```python
from build123d import *

# Parameters (mm, degrees)
SKETCH_1_W          = 20
SKETCH_1_H          = 20
EXTRUDE_1_DEPTH     = 25
SKETCH_2_W          = 20
SKETCH_2_H          = 11.5
CUT_EXTRUDE_1_DEPTH = 5
SKETCH_3_R          = 1.25
CUT_EXTRUDE_2_DEPTH = 25.494897428
SKETCH_4_R          = 1.25
CUT_EXTRUDE_3_DEPTH = 34.541019662
CHAMFER_1_SIZE      = 1
SKETCH_6_R          = 3.5
CUT_EXTRUDE_4_DEPTH = 4


with BuildPart() as part:
    # 草图1 → 凸台-拉伸1 (new body)
    with BuildSketch(Plane(origin=(0, 0, 0), x_dir=(0, 0, -1), z_dir=(1, 0, 0))):
        Rectangle(SKETCH_1_W, SKETCH_1_H)
    extrude(amount=EXTRUDE_1_DEPTH)

    # 草图2 → 切除-拉伸1 (cut)
    with BuildSketch(Plane.ZY):
        Rectangle(SKETCH_2_W, SKETCH_2_H)
    extrude(amount=-CUT_EXTRUDE_1_DEPTH, mode=Mode.SUBTRACT)

    # 草图3 → 切除-拉伸2 (cut, through all)
    with BuildSketch(Plane.ZY.offset(-5)):
        with Locations((-5, 0)):
            Circle(SKETCH_3_R)
        with Locations((5, 0)):
            Circle(SKETCH_3_R)
    extrude(amount=-CUT_EXTRUDE_2_DEPTH, mode=Mode.SUBTRACT)

    # 草图4 → 切除-拉伸3 (cut, through all)
    with BuildSketch(Plane(origin=(0, 10, 0), x_dir=(1, 0, 0), z_dir=(0, 1, 0))):
        with Locations(Location((20, 0, 0), (0, 0, 270))):
            Circle(SKETCH_4_R)
        with Locations(Location((10, 0, 0), (0, 0, 270))):
            Circle(SKETCH_4_R)
    extrude(amount=-CUT_EXTRUDE_3_DEPTH, mode=Mode.SUBTRACT)

    # 倒角1
    chamfer_1_edges = [part.edges().sort_by_distance(p)[0] for p in [
        (25, 0, -10),
        (25, 0, 10),
        (12.5, 10, 10),
        (12.5, 10, -10),
        (12.5, -10, -10),
        (12.5, -10, 10),
    ]]
    chamfer(chamfer_1_edges, length=CHAMFER_1_SIZE)

    # 草图6 → 切除-拉伸4 (cut)
    with BuildSketch(Plane(origin=(25, 0, 0), x_dir=(0, 0, -1), z_dir=(1, 0, 0))):
        with Locations((-5, 0)):
            Circle(SKETCH_6_R)
        with Locations((5, 0)):
            Circle(SKETCH_6_R)
    extrude(amount=-CUT_EXTRUDE_4_DEPTH, mode=Mode.SUBTRACT)


solid = part.part
```
Build history of the part. All positions in model axes, mm. A direction names the side the tool comes from. Coordinates: 2 decimals unless noted, no trailing zeros. Order: outer loops, then holes, each group sorted by start corner. A loop starts at its lowest first (then second) coordinate and runs counter-clockwise, first axis right, second up. Notation, with made-up numbers: (64.25, 11) -> (114.25, 11) arc R14 cw to (114.25, 18) -> close; hole circle Ø11 at (58, 86.5). An arc over 180 degrees is marked (long way). Answer in a Markdown table with one row per item. Add a question column.
Q1. Band-saw the part on A-A, the plane x = 20. List the corners of the cut face in (y, z), then the cut area to 3 significant figures.
Q2. Mould opens along Y. For faces 1 (the face through (12.3, -9.5, -9.5)), 2 (the face through (23.03, 1.05, -8.34)), 3 (the face through (25, 0, 0)) say: +Y half, -Y half, draft (parallel to the pull), parting line (faces both ways), or undercut.
Q3. Band-saw the part on C-C, the plane x = 3. List the corners of the cut face in (y, z).
Q4. Which spindle directions (+Z, -Z, +X, -X, +Y, -Y) get a long thin tool onto all of the face, cutting with end or side? Do faces 4 (the face through (12, 10, 0)), 5 (the face through (5, 0, 0)). Say none if no direction does.
Q5. Drop flat-ended pins along their axis: pin 1 (1.5 mm diameter, centred on y = -2, z = 7, fed in from +X); pin 2 (3 mm diameter, centred on y = 0, z = -5, fed in from +X); pin 3 (2 mm diameter, centred on x = 10, z = 0, fed in from +Y); pin 4 (4 mm diameter, centred on y = -3, z = -4.5, fed in from -X). Give the stop position or say it passes through.
Q6. Wall check: line 1 along X through (y, z) = (2.75, 0); line 2 along Y through (x, z) = (22.25, 5); line 3 along Z through (x, y) = (10.75, -0.25). Give the ranges that are in metal, low to high. Write a range as [from, to].
Q7. Band-saw the part on D-D, the plane z = -5. List the corners of the cut face in (x, y).
Q8. Band-saw the part on B-B, the plane y = 0. List the corners of the cut face in (x, z), then the cut area to 3 significant figures.
Answers follow:
| question | item | result |
|---|---|---|
| 1 | outline | (-10, -9) -> (-9, -10) -> (9, -10) -> (10, -9) -> (10, -1.25) -> (-10, -1.25) -> close; (-10, 1.25) -> (10, 1.25) -> (10, 9) -> (9, 10) -> (-9, 10) -> (-10, 9) -> close; hole circle Ø2.5 at (0, -5); hole circle Ø2.5 at (0, 5) |
| 1 | area | 338 mm^2 |
| 2 | face 1 | -Y half |
| 2 | face 2 | undercut |
| 2 | face 3 | draft |
| 3 | outline | (-10, -9) -> (-9, -10) -> (-5.75, -10) -> (-5.75, 10) -> (-9, 10) -> (-10, 9) -> close; (5.75, -10) -> (9, -10) -> (10, -9) -> (10, 9) -> (9, 10) -> (5.75, 10) -> close |
| 4 | face 4 | +Z, -Z, +X, -X, +Y |
| 4 | face 5 | +Z, -Z, -X |
| 5 | pin 1 | x = 25 |
| 5 | pin 2 | x = 21 |
| 5 | pin 3 | through |
| 5 | pin 4 | x = 5 |
| 6 | line 1 | [5, 8.75], [11.25, 18.75], [21.25, 25] |
| 6 | line 2 | [-10, -3.5], [3.5, 10] |
| 6 | line 3 | [-10, -6.22], [-3.78, -1], [1, 3.78], [6.22, 10] |
| 7 | outline | (0, -10) -> (25, -10) -> (25, -3.5) -> (21, -3.5) -> (21, -1.25) -> (5, -1.25) -> (5, -5.75) -> (0, -5.75) -> close; (0, 5.75) -> (5, 5.75) -> (5, 1.25) -> (21, 1.25) -> (21, 3.5) -> (25, 3.5) -> (25, 10) -> (0, 10) -> close |
| 8 | outline | (5, -10) -> (24, -10) -> (25, -9) -> (25, -8.5) -> (21, -8.5) -> (21, -6.25) -> (5, -6.25) -> close; (5, -3.75) -> (21, -3.75) -> (21, -1.5) -> (25, -1.5) -> (25, 1.5) -> (21, 1.5) -> (21, 3.75) -> (5, 3.75) -> close; (5, 6.25) -> (21, 6.25) -> (21, 8.5) -> (25, 8.5) -> (25, 9) -> (24, 10) -> (5, 10) -> close; hole circle Ø2.5 at (10, 0); hole circle Ø2.5 at (20, 0) |
| 8 | area | 253 mm^2 |
